Work out the finished part from the listing and answer in its coordinate system (mm). A direction names the side the tool comes from. Give positions to 0.01 mm unless a question says otherwise; leave off trailing zeros. Write each loop counter-clockwise with the first axis right and the second up, starting at its lowest first coordinate (ties: lowest second). Pieces come first, ordered by that corner, then holes.
1) Straight lines are drawn through the part: probe 1 along Y at (x, z) = (0, -9.5); probe 2 along Y at (x, z) = (0, 1.8); probe 3 along X at (y, z) = (1, -5.5). For each, find the intervals that lie inside material, in ascending order.
2) A tool of negligible diameter and unlimited length cuts with its end or side. For faces 1 (the face through (-10, -33, 0)), 2 (the face through (42.397, 13.352, 1.252)), from which of +Z, -Z, +X, -X, +Y, -Y can it reach the whole face along a straight path? Write none if from no direction.
3) Given pin 1 Ø4 at (y, z) = (-22, -5) entering from +X; pin 2 Ø8 at (y, z) = (9, -4.5) entering from -X; pin 3 Ø1 at (x, z) = (23.5, -10.5) entering from -Y, each flat-ended and moving along its own axis, determine where each tip first touches the part or whether it passes through.
4) Find section C-C (z = -7.5). Determine the outline of the cut face in (x, y).
5) Find section A-A (y = 0). Determine the outline of the cut face in (x, z).
```python
from build123d import *

# Parameters (mm, degrees)
F0_R          = 44.45
F0_R_2        = 34.163
F1_DEPTH      = 2.54
F0_R_3        = 33.401
F2_DEPTH      = 2.54
F2_DEPTH_BACK = 12.7


with BuildPart() as f1:
    # F0 (on Top) → F1 (new body)
    with BuildSketch(Plane.XY):
        Circle(F0_R)
        Circle(F0_R_2, mode=Mode.SUBTRACT)
    extrude(amount=F1_DEPTH)

    # F0 (on Top) → F2 (join, two sides)
    with BuildSketch(Plane.XY) as f2_sk:
        Circle(F0_R_2)
        Circle(F0_R_3, mode=Mode.SUBTRACT)
    extrude(amount=F2_DEPTH)
    extrude(f2_sk.sketch, amount=-F2_DEPTH_BACK)


solid = f1.part
```
Results:
1. probe 1: y = -34.16 to -33.4, 33.4 to 34.16
1. probe 2: y = -44.45 to -33.4, 33.4 to 44.45
1. probe 3: x = -34.15 to -33.39, 33.39 to 34.15
2. face 1: -Z
2. face 2: +Z, -Z
3. pin 1: stops at x = 27.7
3. pin 2: stops at x = -33.8
3. pin 3: stops at y = -25.26
4. outline: circle Ø68.33 at (0, 0); hole circle Ø66.8 at (0, 0)
5. outline: (-44.45, 0) - (-34.16, 0) - (-34.16, -12.7) - (-33.4, -12.7) - (-33.4, 2.54) - (-44.45, 2.54) - close; (33.4, -12.7) - (34.16, -12.7) - (34.16, 0) - (44.45, 0) - (44.45, 2.54) - (33.4, 2.54) - close
